Geometry: final body of the model. Coordinates: model frame, mm. A direction names the side the tool comes from. Give positions to 0.01 mm unless a question says otherwise; leave off trailing zeros. Answer in a Markdown table with one row per item. Add a question column.
Q1. Line query: line 1 along X through (y, z) = (-255.5, -6); line 2 along Z through (x, y) = (0, -350). Output: solid intervals per line, ascending. Write a range as from..to.
Q2. Contact query for a flat-ended pin moving along its axis: P1, Ø2, axis at x = 1, y = -256, coming from the -Z side. Output: stop coordinate, or through.
Q3. Pull-direction query (X, two-part tool) for faces 1 (the face through (0, -269, -10)), 2 (the face through (-12, -269, -20)), 3 (the face through (-10, -269, 0)), 4 (the face through (20, -269, 11)); classes: +X half, -X half, draft (parallel to the pull), parting line (faces both ways), or undercut.
Q4. Set-up query: faces 5 (the face through (-12, -269, 20)), 6 (the face through (0, -269, 10)). Return all of +Z, -Z, +X, -X, +Y, -Y with unobstructed straight access to the full face (end or side cutting, diameter ignored); none if empty.
from build123d import *

# Parameters (mm, degrees)
F0_W     = 40
F0_H     = 40
F1_DEPTH = 545
F2_W     = 5
F2_H     = 10
F2_W_2   = 10
F2_H_2   = 5
F2_R     = 3
F3_DEPTH = 545.001
F4_R     = 2


with BuildPart() as f1:
    # F0 (on Front) → F1 (new body)
    with BuildSketch(Plane.XZ):
        Rectangle(F0_W, F0_H)
    extrude(amount=F1_DEPTH)

    # F2 (on face) → F3 (cut, through all)
    with BuildSketch(Plane(origin=(0, 0, 0), x_dir=(-1, 0, 0), z_dir=(0, 1, 0))):
        with Locations((-17.5, 0)):
            Rectangle(F2_W, F2_H)
        Polygon((-15, 8), (-15, 5), (-15, -5), (-15, -8), (-10, -8), (-10, 8), align=None)
        Polygon((5, 15), (-5, 15), (-8, 15), (-8, 10), (8, 10), (8, 15), align=None)
        with Locations((0, 17.5)):
            Rectangle(F2_W_2, F2_H_2)
        Polygon((15, -5), (15, 5), (15, 8), (10, 8), (10, -8), (15, -8), align=None)
        with Locations((17.5, 0)):
            Rectangle(F2_W, F2_H)
        Circle(F2_R)
        Polygon((-8, -15), (-5, -15), (5, -15), (8, -15), (8, -10), (-8, -10), align=None)
        with Locations((0, -17.5)):
            Rectangle(F2_W_2, F2_H_2)
    extrude(amount=-F3_DEPTH, mode=Mode.SUBTRACT)

    # F4
    f4_edges = [f1.edges().sort_by_distance(p)[0] for p in [
        (20, -272.5, 20),
        (-20, -272.5, 20),
        (20, -272.5, -20),
        (-20, -272.5, -20),
    ]]
    fillet(f4_edges, radius=F4_R)


solid = f1.part
Completed:
| question | item | result |
|---|---|---|
| 1 | line 1 | x = -20..-15, -10..10, 15..20 |
| 1 | line 2 | z = -10..-3, 3..10 |
| 2 | P1 | stops at z = -10 |
| 3 | face 1 | undercut |
| 3 | face 2 | draft |
| 3 | face 3 | undercut |
| 3 | face 4 | +X half |
| 4 | face 5 | +Z, +X, -X, +Y, -Y |
| 4 | face 6 | +Y, -Y |
